Could you check a few things on this drawing? It's one solid part, dimensions in mm from its lowest x, y, z. A direction names the side the tool comes from. Give positions to 0.01 mm unless a question says otherwise; leave off trailing zeros. Loops run counter-clockwise (first coordinate to the right, second up) from the corner with the lowest first, then second, coordinate; pieces in that order, holes last. Notation, with made-up numbers: (-23.75, 5) - (35.25, 5) arc R17 cw to (35.25, 12) - close; hole circle Ø2 at (-20.5, -28). An arc over 180 degrees is marked (long way). Write item = value, one per line.
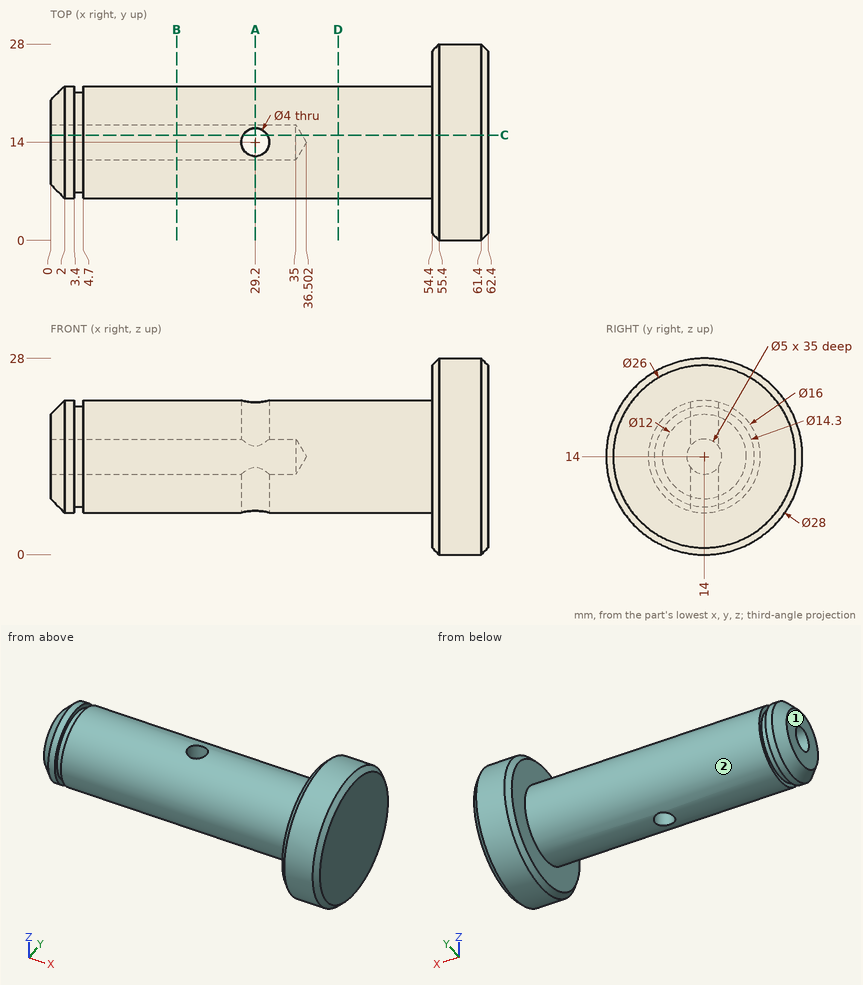
Q1. Which directions (+Z, -Z, +X, -X, +Y, -Y) give clear straight access to the entire face, cutting with the end or side of a thin tool? Please do the marked faces 1 and 2.
Output:
face_1 = +Z, -Z, -X, +Y, -Y
face_2 = -X
Q2. Imagine slicing it at A-A, the plane x = 29.2. Write out the boundary of the cut face in (y, z), then the cut area to 3 significant figures.
Output:
outline = (12, 6.25) - (12, 12.5) arc R2.5 cw to (12, 15.5) - (12, 21.75) arc R8 ccw to start; (16, 6.25) arc R8 ccw to (16, 21.75) - (16, 15.5) arc R2.5 cw to (16, 12.5) - close
area = 136 mm2
Q3. For pin 1 (4 mm diameter, centred on x = 11.5, y = 15, fed in from +Z); pin 2 (5 mm diameter, centred on x = 14, y = 10.5, fed in from +Z); pin 3 (5 mm diameter, centred on x = 37.5, y = 13, fed in from -Z), each with a flat end and sliding along its axis, tell me the tip position at first contact or that it passes through.
Output:
pin_1 = 22
pin_2 = 21.94
pin_3 = 6
Q4. I need wall thicknesses on L1, parallel to X at y = 14, z = 19.75; L2, parallel to Z at x = 26, y = 14; L3, parallel to X at y = 24.25, z = 12. Which ranges of each line are inside material? Lowest first, please.
Output:
L1 = 0 to 27.2, 31.2 to 62.4
L2 = 6 to 11.5, 16.5 to 22
L3 = 54.4 to 62.4
Q5. Imagine slicing it at C-C, the plane y = 15. Give the number of separate pieces and of enclosed holes in the cut face, then the cut area to 3 significant figures.
Output:
separate_pieces = 3
enclosed_holes = 0
area = 877 mm2
Q6. Imagine slicing it at B-B, the plane x = 18. Write out the boundary of the cut face in (y, z).
Output:
outline = circle Ø16 at (14, 14); hole circle Ø5 at (14, 14)
Q7. Imagine slicing it at D-D, the plane x = 41. Write out the boundary of the cut face in (y, z).
Output:
outline = circle Ø16 at (14, 14)
